The listing builds one solid part. Answer for the finished solid, in the listing's coordinates (mm). Give positions to 0.01 mm unless a question says otherwise; leave off trailing zeros. Loops run counter-clockwise (first coordinate to the right, second up) from the corner with the lowest first, then second, coordinate; pieces in that order, holes last.
Item 1: Consider line 1 along X through (y, z) = (-2.3, -24.75); line 2 along Z through (x, y) = (31.25, -1.9); line 3 along Y through (x, z) = (16.5, -27.5). Determine where each line is inside the solid, lowest interval first.
Item 2: Section A-A, the plane x = 33.25 is taken. Give the vertices of the cut face in (y, z) (3 decimals).
Item 3: Section B-B, the plane z = -20 is taken. Give the vertices of the cut face in (x, y), and give its area (3 significant figures).
Item 4: This flat-tipped pin is pushed along its axis until it touches: pin 1 Ø2 at (x, z) = (22.5, -19.5) entering from +Y. Where does it stop, or does it pass through?
Item 5: The mould has two halves that part along Z. Classify faces 1 (the face through (24.86, -2.777, -19.037)), 2 (the face through (25, -2.353, -25)), 3 (the face through (35, -2, -25)), 4 (the face through (24.86, -2.767, -31.011)): pulls with the +Z half, pulls with the -Z half, needs draft (parallel to the pull), parting line crosses it, or undercut.
Item 6: Section C-C, the plane y = -2.8 is taken. Give the vertices of the cut face in (x, z), and give its area (3 significant figures).
from build123d import *

# Parameters (mm, degrees)
EXTRUDE_1_DEPTH     = 50
SKETCH_2_W          = 47.752029062465894
SKETCH_2_H          = 35.88941973747437
CUT_EXTRUDE_1_DEPTH = 2
FILLET_1_R          = 1
SCALE_1_SCALE       = 0.4


with BuildPart() as part:
    # 草图1 → 凸台-拉伸1 (new body)
    with BuildSketch(Plane(origin=(0, 0, 0), x_dir=(0, 0, -1), z_dir=(1, 0, 0))):
        with BuildLine():
            Line((6.066042211617314, 0), (43.933957788382685, 0))
            ThreePointArc((43.933957788382685, 0), (44.92401323811772, -0.85932233137432), (44.212515173340435, -1.9604195871000956))
            ThreePointArc((44.212515173340435, -1.9604195871000956), (39.96661362209007, -3.046903416934029), (35.66027972203156, -3.861529365825664))
            Line((35.66027972203156, -3.861529365825664), (14.339720277968421, -3.861529365825664))
            ThreePointArc((14.339720277968421, -3.861529365825664), (10.03338637790992, -3.046903416934029), (5.787484826659573, -1.9604195871000956))
            ThreePointArc((5.787484826659573, -1.9604195871000956), (5.075986761882271, -0.8593223313743236), (6.066042211617314, 0))
        make_face()
    extrude(amount=EXTRUDE_1_DEPTH)

    # 草图2 → 切除-拉伸1 (cut)
    with BuildSketch(Plane(origin=(0, 0, 0), x_dir=(1, 0, 0), z_dir=(0, 1, 0))):
        with Locations((25, 25.000000000000007)):
            Rectangle(SKETCH_2_W, SKETCH_2_H)
    extrude(amount=-CUT_EXTRUDE_1_DEPTH, mode=Mode.SUBTRACT)

    # 圆角1
    # the kernel refuses this fillet: 1 mm, written as the material it takes off along each edge
    with BuildSketch(Plane(origin=(1.1239854687670539, 0, -7.055290131262825), x_dir=(-1, 0, 0), z_dir=(0, 0, -1))) as fillet_1_piece_1:
        with BuildLine():
            CenterArc((FILLET_1_R, -FILLET_1_R), FILLET_1_R, 90, 90)
            Line((0, -FILLET_1_R), (-FILLET_1_R * 0.02, -FILLET_1_R))
            Line((-FILLET_1_R * 0.02, -FILLET_1_R), (-FILLET_1_R * 0.02, FILLET_1_R * 0.02))
            Line((-FILLET_1_R * 0.02, FILLET_1_R * 0.02), (FILLET_1_R, FILLET_1_R * 0.02))
            Line((FILLET_1_R, FILLET_1_R * 0.02), (FILLET_1_R, 0))
        make_face()
    extrude(amount=35.88941973747437, mode=Mode.SUBTRACT)
    with BuildSketch(Plane(origin=(48.87601453123295, 0, -7.055290131262825), x_dir=(0, 0, 1), z_dir=(-1, 0, 0))) as fillet_1_piece_2:
        with BuildLine():
            CenterArc((FILLET_1_R, -FILLET_1_R), FILLET_1_R, 90, 90)
            Line((0, -FILLET_1_R), (-FILLET_1_R * 0.02, -FILLET_1_R))
            Line((-FILLET_1_R * 0.02, -FILLET_1_R), (-FILLET_1_R * 0.02, FILLET_1_R * 0.02))
            Line((-FILLET_1_R * 0.02, FILLET_1_R * 0.02), (FILLET_1_R, FILLET_1_R * 0.02))
            Line((FILLET_1_R, FILLET_1_R * 0.02), (FILLET_1_R, 0))
        make_face()
    extrude(amount=47.752029062465894, mode=Mode.SUBTRACT)
    with BuildSketch(Plane(origin=(48.87601453123295, 0, -42.94470986873719), x_dir=(1, 0, 0), z_dir=(0, 0, 1))) as fillet_1_piece_3:
        with BuildLine():
            CenterArc((FILLET_1_R, -FILLET_1_R), FILLET_1_R, 90, 90)
            Line((0, -FILLET_1_R), (-FILLET_1_R * 0.02, -FILLET_1_R))
            Line((-FILLET_1_R * 0.02, -FILLET_1_R), (-FILLET_1_R * 0.02, FILLET_1_R * 0.02))
            Line((-FILLET_1_R * 0.02, FILLET_1_R * 0.02), (FILLET_1_R, FILLET_1_R * 0.02))
            Line((FILLET_1_R, FILLET_1_R * 0.02), (FILLET_1_R, 0))
        make_face()
    extrude(amount=35.88941973747437, mode=Mode.SUBTRACT)
    with BuildSketch(Plane(origin=(1.1239854687670539, 0, -42.94470986873719), x_dir=(0, 0, -1), z_dir=(1, 0, 0))) as fillet_1_piece_4:
        with BuildLine():
            CenterArc((FILLET_1_R, -FILLET_1_R), FILLET_1_R, 90, 90)
            Line((0, -FILLET_1_R), (-FILLET_1_R * 0.02, -FILLET_1_R))
            Line((-FILLET_1_R * 0.02, -FILLET_1_R), (-FILLET_1_R * 0.02, FILLET_1_R * 0.02))
            Line((-FILLET_1_R * 0.02, FILLET_1_R * 0.02), (FILLET_1_R, FILLET_1_R * 0.02))
            Line((FILLET_1_R, FILLET_1_R * 0.02), (FILLET_1_R, 0))
        make_face()
    extrude(amount=47.752029062465894, mode=Mode.SUBTRACT)
    with BuildSketch(Plane(origin=(1.1239854687670539, 0, -4.555290131262826), x_dir=(-1, 0, 0), z_dir=(0, 0, -1))) as fillet_1_piece_5a_section:
        with BuildLine():
            CenterArc((FILLET_1_R, -FILLET_1_R), FILLET_1_R, 90, 90)
            Line((0, -FILLET_1_R), (-FILLET_1_R * 0.02, -FILLET_1_R))
            Line((-FILLET_1_R * 0.02, -FILLET_1_R), (-FILLET_1_R * 0.02, FILLET_1_R * 0.02))
            Line((-FILLET_1_R * 0.02, FILLET_1_R * 0.02), (FILLET_1_R, FILLET_1_R * 0.02))
            Line((FILLET_1_R, FILLET_1_R * 0.02), (FILLET_1_R, 0))
        make_face()
    fillet_1_piece_5a = extrude(amount=38.38941973747437, mode=Mode.PRIVATE)
    fillet_1_piece_5a = split(fillet_1_piece_5a, bisect_by=Plane(origin=(0.8975903545002311, -0.2263951142668261, -7.055290131262825), z_dir=(0, 0, 1)), keep=Keep.TOP, mode=Mode.PRIVATE)
    with BuildSketch(Plane(origin=(48.87601453123295, 0, -7.055290131262825), x_dir=(0, 0, 1), z_dir=(-1, 0, 0))) as fillet_1_piece_5b_section:
        with BuildLine():
            CenterArc((FILLET_1_R, -FILLET_1_R), FILLET_1_R, 90, 90)
            Line((0, -FILLET_1_R), (-FILLET_1_R * 0.02, -FILLET_1_R))
            Line((-FILLET_1_R * 0.02, -FILLET_1_R), (-FILLET_1_R * 0.02, FILLET_1_R * 0.02))
            Line((-FILLET_1_R * 0.02, FILLET_1_R * 0.02), (FILLET_1_R, FILLET_1_R * 0.02))
            Line((FILLET_1_R, FILLET_1_R * 0.02), (FILLET_1_R, 0))
        make_face()
    fillet_1_piece_5b = extrude(amount=50.252029062465894, mode=Mode.PRIVATE)
    fillet_1_piece_5b = split(fillet_1_piece_5b, bisect_by=Plane(origin=(1.1239854687670539, -0.22639511426682482, -6.828895016995999), z_dir=(-1, 0, 0)), keep=Keep.TOP, mode=Mode.PRIVATE)
    fillet_1_piece_5 = fillet_1_piece_5a & fillet_1_piece_5b
    add(fillet_1_piece_5, mode=Mode.SUBTRACT)
    with BuildSketch(Plane(origin=(1.1239854687670539, 0, -7.055290131262825), x_dir=(-1, 0, 0), z_dir=(0, 0, -1))) as fillet_1_piece_6a_section:
        with BuildLine():
            CenterArc((FILLET_1_R, -FILLET_1_R), FILLET_1_R, 90, 90)
            Line((0, -FILLET_1_R), (-FILLET_1_R * 0.02, -FILLET_1_R))
            Line((-FILLET_1_R * 0.02, -FILLET_1_R), (-FILLET_1_R * 0.02, FILLET_1_R * 0.02))
            Line((-FILLET_1_R * 0.02, FILLET_1_R * 0.02), (FILLET_1_R, FILLET_1_R * 0.02))
            Line((FILLET_1_R, FILLET_1_R * 0.02), (FILLET_1_R, 0))
        make_face()
    fillet_1_piece_6a = extrude(amount=38.38941973747437, mode=Mode.PRIVATE)
    fillet_1_piece_6a = split(fillet_1_piece_6a, bisect_by=Plane(origin=(0.8975903545002285, -0.22639511426682538, -42.94470986873719), z_dir=(0, 0, -1)), keep=Keep.TOP, mode=Mode.PRIVATE)
    with BuildSketch(Plane(origin=(-1.3760145312329461, 0, -42.94470986873719), x_dir=(0, 0, -1), z_dir=(1, 0, 0))) as fillet_1_piece_6b_section:
        with BuildLine():
            CenterArc((FILLET_1_R, -FILLET_1_R), FILLET_1_R, 90, 90)
            Line((0, -FILLET_1_R), (-FILLET_1_R * 0.02, -FILLET_1_R))
            Line((-FILLET_1_R * 0.02, -FILLET_1_R), (-FILLET_1_R * 0.02, FILLET_1_R * 0.02))
            Line((-FILLET_1_R * 0.02, FILLET_1_R * 0.02), (FILLET_1_R, FILLET_1_R * 0.02))
            Line((FILLET_1_R, FILLET_1_R * 0.02), (FILLET_1_R, 0))
        make_face()
    fillet_1_piece_6b = extrude(amount=50.252029062465894, mode=Mode.PRIVATE)
    fillet_1_piece_6b = split(fillet_1_piece_6b, bisect_by=Plane(origin=(1.1239854687670539, -0.22639511426682907, -43.171104983004014), z_dir=(-1, 0, 0)), keep=Keep.TOP, mode=Mode.PRIVATE)
    fillet_1_piece_6 = fillet_1_piece_6a & fillet_1_piece_6b
    add(fillet_1_piece_6, mode=Mode.SUBTRACT)
    with BuildSketch(Plane(origin=(51.37601453123295, 0, -7.055290131262825), x_dir=(0, 0, 1), z_dir=(-1, 0, 0))) as fillet_1_piece_7a_section:
        with BuildLine():
            CenterArc((FILLET_1_R, -FILLET_1_R), FILLET_1_R, 90, 90)
            Line((0, -FILLET_1_R), (-FILLET_1_R * 0.02, -FILLET_1_R))
            Line((-FILLET_1_R * 0.02, -FILLET_1_R), (-FILLET_1_R * 0.02, FILLET_1_R * 0.02))
            Line((-FILLET_1_R * 0.02, FILLET_1_R * 0.02), (FILLET_1_R, FILLET_1_R * 0.02))
            Line((FILLET_1_R, FILLET_1_R * 0.02), (FILLET_1_R, 0))
        make_face()
    fillet_1_piece_7a = extrude(amount=50.252029062465894, mode=Mode.PRIVATE)
    fillet_1_piece_7a = split(fillet_1_piece_7a, bisect_by=Plane(origin=(48.87601453123295, -0.22639511426682557, -6.828895016996), z_dir=(1, 0, 0)), keep=Keep.TOP, mode=Mode.PRIVATE)
    with BuildSketch(Plane(origin=(48.87601453123295, 0, -42.94470986873719), x_dir=(1, 0, 0), z_dir=(0, 0, 1))) as fillet_1_piece_7b_section:
        with BuildLine():
            CenterArc((FILLET_1_R, -FILLET_1_R), FILLET_1_R, 90, 90)
            Line((0, -FILLET_1_R), (-FILLET_1_R * 0.02, -FILLET_1_R))
            Line((-FILLET_1_R * 0.02, -FILLET_1_R), (-FILLET_1_R * 0.02, FILLET_1_R * 0.02))
            Line((-FILLET_1_R * 0.02, FILLET_1_R * 0.02), (FILLET_1_R, FILLET_1_R * 0.02))
            Line((FILLET_1_R, FILLET_1_R * 0.02), (FILLET_1_R, 0))
        make_face()
    fillet_1_piece_7b = extrude(amount=38.38941973747437, mode=Mode.PRIVATE)
    fillet_1_piece_7b = split(fillet_1_piece_7b, bisect_by=Plane(origin=(49.10240964549977, -0.22639511426682904, -7.055290131262825), z_dir=(0, 0, 1)), keep=Keep.TOP, mode=Mode.PRIVATE)
    fillet_1_piece_7 = fillet_1_piece_7a & fillet_1_piece_7b
    add(fillet_1_piece_7, mode=Mode.SUBTRACT)
    with BuildSketch(Plane(origin=(48.87601453123295, 0, -45.44470986873719), x_dir=(1, 0, 0), z_dir=(0, 0, 1))) as fillet_1_piece_8a_section:
        with BuildLine():
            CenterArc((FILLET_1_R, -FILLET_1_R), FILLET_1_R, 90, 90)
            Line((0, -FILLET_1_R), (-FILLET_1_R * 0.02, -FILLET_1_R))
            Line((-FILLET_1_R * 0.02, -FILLET_1_R), (-FILLET_1_R * 0.02, FILLET_1_R * 0.02))
            Line((-FILLET_1_R * 0.02, FILLET_1_R * 0.02), (FILLET_1_R, FILLET_1_R * 0.02))
            Line((FILLET_1_R, FILLET_1_R * 0.02), (FILLET_1_R, 0))
        make_face()
    fillet_1_piece_8a = extrude(amount=38.38941973747437, mode=Mode.PRIVATE)
    fillet_1_piece_8a = split(fillet_1_piece_8a, bisect_by=Plane(origin=(49.10240964549977, -0.2263951142668292, -42.94470986873719), z_dir=(0, 0, -1)), keep=Keep.TOP, mode=Mode.PRIVATE)
    with BuildSketch(Plane(origin=(1.1239854687670539, 0, -42.94470986873719), x_dir=(0, 0, -1), z_dir=(1, 0, 0))) as fillet_1_piece_8b_section:
        with BuildLine():
            CenterArc((FILLET_1_R, -FILLET_1_R), FILLET_1_R, 90, 90)
            Line((0, -FILLET_1_R), (-FILLET_1_R * 0.02, -FILLET_1_R))
            Line((-FILLET_1_R * 0.02, -FILLET_1_R), (-FILLET_1_R * 0.02, FILLET_1_R * 0.02))
            Line((-FILLET_1_R * 0.02, FILLET_1_R * 0.02), (FILLET_1_R, FILLET_1_R * 0.02))
            Line((FILLET_1_R, FILLET_1_R * 0.02), (FILLET_1_R, 0))
        make_face()
    fillet_1_piece_8b = extrude(amount=50.252029062465894, mode=Mode.PRIVATE)
    fillet_1_piece_8b = split(fillet_1_piece_8b, bisect_by=Plane(origin=(48.87601453123295, -0.22639511426682885, -43.17110498300402), z_dir=(1, 0, 0)), keep=Keep.TOP, mode=Mode.PRIVATE)
    fillet_1_piece_8 = fillet_1_piece_8a & fillet_1_piece_8b
    add(fillet_1_piece_8, mode=Mode.SUBTRACT)


with BuildPart() as part_1:
    # 缩放比例1: scaled about (25, -2.588659759, -25)
    add(part.part.scale(SCALE_1_SCALE).moved(Location((15, -1.5531958554, -15))))


solid = part_1.part
Worked answers:
1. line 1: x = 15 to 15.45, 34.55 to 35
1. line 2: z = -32.97 to -32.18, -17.82 to -17.03
1. line 3: y = -3.1 to -2.35
2. outline: (-3.098, -29.264) arc R27.589 ccw to (-2.337, -32.685) arc R0.4 ccw to (-1.553, -32.576) arc R0.4 ccw to (-1.953, -32.178) - (-2.353, -32.178) - (-2.353, -17.822) - (-1.953, -17.822) arc R0.4 ccw to (-1.553, -17.424) arc R0.4 ccw to (-2.337, -17.315) arc R27.589 ccw to (-3.098, -20.736) - close
3. outline: (15, -2.97) - (35, -2.97) - (35, -1.55) - (34.95, -1.55) arc R0.4 ccw to (34.55, -1.95) - (34.55, -2.35) - (15.45, -2.35) - (15.45, -1.95) arc R0.4 ccw to (15.05, -1.55) - (15, -1.55) - close
3. area: 13.0 mm2
4. pin 1: stops at y = -2.35
5. face 1: pulls with the +Z half
5. face 2: undercut
5. face 3: needs draft
5. face 4: pulls with the -Z half
6. outline: (15, -30.86) - (35, -30.86) - (35, -19.14) - (15, -19.14) - close
6. area: 234 mm2
